from build123d import *

# Parameters (mm, degrees)
SKETCH1_W           = 100
SKETCH1_H           = 60
SKETCH1_W_2         = 97
SKETCH1_H_2         = 57
BOSS_EXTRUDE1_DEPTH = 20
SKETCH2_W           = 100
SKETCH2_H           = 60
BOSS_EXTRUDE2_DEPTH = 1.5
SKETCH3_W           = 10
SKETCH3_H           = 2
BOSS_EXTRUDE3_DEPTH = 100
SKETCH4_R           = 1.55
CUT_EXTRUDE1_DEPTH  = 2
SKETCH5_R           = 4
CUT_EXTRUDE2_DEPTH  = 3


with BuildPart() as part:
    # Sketch1 → Boss-Extrude1 (new body)
    with BuildSketch(Plane(origin=(0, 0, 0), x_dir=(1, 0, 0), z_dir=(0, 1, 0))):
        Rectangle(SKETCH1_W, SKETCH1_H)
        Rectangle(SKETCH1_W_2, SKETCH1_H_2, mode=Mode.SUBTRACT)
    extrude(amount=BOSS_EXTRUDE1_DEPTH)

    # Sketch2 → Boss-Extrude2 (add)
    with BuildSketch(Plane(origin=(0, 20, 0), x_dir=(1, 0, 0), z_dir=(0, 1, 0))):
        Rectangle(SKETCH2_W, SKETCH2_H)
    extrude(amount=BOSS_EXTRUDE2_DEPTH)

    # Sketch3 → Boss-Extrude3 (add)
    with BuildSketch(Plane(origin=(50, 0, 0), x_dir=(0, 0, -1), z_dir=(1, 0, 0))):
        with Locations((-35, 1)):
            Rectangle(SKETCH3_W, SKETCH3_H)
        with Locations((35, 1)):
            Rectangle(SKETCH3_W, SKETCH3_H)
    extrude(amount=-BOSS_EXTRUDE3_DEPTH)

    # Sketch4 → Cut-Extrude1 (cut)
    with BuildSketch(Plane.XZ):
        with Locations(Location((-45, 35, 0), (0, 0, 270))):
            Circle(SKETCH4_R)
        with Locations(Location((45, 35, 0), (0, 0, 270))):
            Circle(SKETCH4_R)
        with Locations(Location((45, -35, 0), (0, 0, 270))):
            Circle(SKETCH4_R)
        with Locations(Location((-45, -35, 0), (0, 0, 270))):
            Circle(SKETCH4_R)
        with Locations(Location((5, 35, 0), (0, 0, 270))):
            Circle(SKETCH4_R)
        with Locations(Location((5, -35, 0), (0, 0, 270))):
            Circle(SKETCH4_R)
    extrude(amount=-CUT_EXTRUDE1_DEPTH, mode=Mode.SUBTRACT)

    # Sketch5 → Cut-Extrude2 (cut)
    with BuildSketch(Plane(origin=(0, 21.5, 0), x_dir=(1, 0, 0), z_dir=(0, 1, 0))):
        with Locations(Location((12.44, -9.95, 0), (0, 0, 270))):
            Circle(SKETCH5_R)
    extrude(amount=-CUT_EXTRUDE2_DEPTH, mode=Mode.SUBTRACT)


solid = part.part
Input: part model. Units: mm. Frame: model coordinates. A direction names the side the tool comes from. Coordinates: 2 decimals unless noted, no trailing zeros. Loops run counter-clockwise (first coordinate to the right, second up) from the corner with the lowest first, then second, coordinate; pieces in that order, holes last. Notation, with made-up numbers: (53, 31) -> (59, 31) arc R19 ccw to (59, 40) -> close; hole circle Ø4 at (-11.75, 52). An arc over 180 degrees is marked (long way). Write each question's results on one line, items separated by ' | '. Start each with the question number.
Q1. Pull-direction query (X, two-part tool) for faces 1 (the flat face through (-50, 11, 1)), 2 (the cylindrical face through (13.641, 20.76, 13.765)), 3 (the flat face through (1, 1, -40)); classes: released by +X, released by -X, zero draft, split by the parting line, or undercut.
Q2. Section A-A, the plane x = 45. Return the cut outline in (y, z).
Q3. Pin query (flat end, axial travel): pin 1 (10 mm diameter, centred on x = -22.5, y = 14, fed in from +Z); pin 2 (8 mm diameter, centred on x = 8, z = -35.5, fed in from +Y); pin 3 (3 mm diameter, centred on x = 45, z = -35, fed in from +Y); pin 4 (6 mm diameter, centred on x = 6, z = 10.5, fed in from -Y). Return the tip coordinate at first contact, or that it passes through.
Q4. Section D-D, the plane z = -35. Return the cut outline in (x, y), plus the area to 3 significant figures.
Q5. Reachability of faces 4 (the flat face through (1, 2, -35)), 5 (the flat face through (-1, 12, 30)), 6 (the cylindrical face through (43.625, 0.986, -35.715)), 7 (the flat face through (-48.5, 10, 0)) from +Z, -Z, +X, -X, +Y, -Y: full face, straight path, thin tool, end or side. Return the list, or none.
Q6. Section C-C, the plane x = 12.44. Return the cut outline in (y, z).
Q7. Section B-B, the plane y = 11.5. Return the cut outline in (x, z), plus the area to 3 significant figures.
Q8. Ray query, line 1 (X direction, y = 1.15, z = 35); line 2 (Z direction, x = -31.5, y = 19.5); line 3 (X direction, y = 8.25, z = -11.5). Return the intervals inside material, ascending. Write a range as from..to.
Found:
1) face 1: released by -X | face 2: undercut | face 3: zero draft
2) outline: (0, -40) -> (2, -40) -> (2, -36.55) -> (0, -36.55) -> close; (0, -33.45) -> (2, -33.45) -> (2, -30) -> (21.5, -30) -> (21.5, 30) -> (2, 30) -> (2, 33.45) -> (0, 33.45) -> (0, 28.5) -> (20, 28.5) -> (20, -28.5) -> (0, -28.5) -> close; (0, 36.55) -> (2, 36.55) -> (2, 40) -> (0, 40) -> close
3) pin 1: z = 30 | pin 2: y = 2 | pin 3: through | pin 4: y = 20
4) outline: (-50, 0) -> (-46.55, 0) -> (-46.55, 2) -> (-50, 2) -> close; (-43.45, 0) -> (3.45, 0) -> (3.45, 2) -> (-43.45, 2) -> close; (6.55, 0) -> (43.45, 0) -> (43.45, 2) -> (6.55, 2) -> close; (46.55, 0) -> (50, 0) -> (50, 2) -> (46.55, 2) -> close | area: 181 mm2
5) face 4: -Z, +X, -X, +Y | face 5: +Z, +X, -X, +Y | face 6: +Y, -Y | face 7: -Y
6) outline: (0, -40) -> (2, -40) -> (2, -30) -> (21.5, -30) -> (21.5, 5.95) -> (20, 5.95) -> (20, -28.5) -> (0, -28.5) -> close; (0, 28.5) -> (20, 28.5) -> (20, 13.95) -> (21.5, 13.95) -> (21.5, 30) -> (2, 30) -> (2, 40) -> (0, 40) -> close
7) outline: (-50, -30) -> (50, -30) -> (50, 30) -> (-50, 30) -> close; hole (-48.5, -28.5) -> (48.5, -28.5) -> (48.5, 28.5) -> (-48.5, 28.5) -> close | area: 471 mm2
8) line 1: -50..-46.55, -43.45..3.45, 6.55..43.45, 46.55..50 | line 2: -30..-28.5, 28.5..30 | line 3: -50..-48.5, 48.5..50
